```python
from build123d import *

# Parameters (mm, degrees)
SKETCH_W     = 20
SKETCH_H     = 10
SKETCH_R     = 1.25
PAD_DEPTH    = 6.5
SKETCH001_W  = 19
SKETCH001_H  = 4
PAD001_DEPTH = 0.1
SKETCH002_W  = 4
SKETCH002_H  = 0.1
PAD002_DEPTH = 5
FILLET_R     = 1.99
SKETCH003_R  = 2.5
PAD003_DEPTH = 3.8
SKETCH004_W  = 0.5
SKETCH004_H  = 3
PAD004_DEPTH = 4
FILLET001_R  = 1.49


with BuildPart() as part:
    # Sketch → Pad (new body)
    with BuildSketch(Plane.XZ):
        with Locations((10, 5)):
            Rectangle(SKETCH_W, SKETCH_H)
        with Locations((5, 2.5)):
            Circle(SKETCH_R, mode=Mode.SUBTRACT)
        with Locations((15, 2.5)):
            Circle(SKETCH_R, mode=Mode.SUBTRACT)
    extrude(amount=PAD_DEPTH)

    # Sketch001 (on Face3 of Pad) → Pad001 (join)
    with BuildSketch(Plane(origin=(2.5, 1.5, 10), x_dir=(-0.965926, 0, -0.258819), z_dir=(-0.258819, 0, 0.965926))):
        with Locations((-9.5, 4.728916)):
            Rectangle(SKETCH001_W, SKETCH001_H)
    extrude(amount=-PAD001_DEPTH)

    # Sketch002 (on Face12 of Pad001) → Pad002 (join)
    with BuildSketch(Plane(origin=(-2.332532, 0, 8.705127), x_dir=(-0.965926, 0, -0.258819), z_dir=(-0.258819, 0, 0.965926))):
        with Locations((-22.003005, 5.178916)):
            Rectangle(SKETCH002_W, SKETCH002_H)
        with Locations((-22.003005, 1.278916)):
            Rectangle(SKETCH002_W, SKETCH002_H)
    extrude(amount=PAD002_DEPTH)

    # Fillet
    fillet_edges = [part.edges().sort_by_distance(p)[0] for p in [
        (19.558495, -5.178916, 19.747191),
        (15.694792, -5.178916, 18.711915),
        (15.694792, -1.278916, 18.711915),
        (19.558495, -1.278916, 19.747191),
    ]]
    fillet(fillet_edges, radius=FILLET_R)

    # Sketch003 (on Face5 of Fillet) → Pad003 (join)
    with BuildSketch(Plane.XZ.offset(1.328916)):
        with Locations((18.132034, 17.304772)):
            Circle(SKETCH003_R)
    extrude(amount=PAD003_DEPTH)

    # Sketch004 (on Face24 of Pad003) → Pad004 (join)
    with BuildSketch(Plane(origin=(0, 0, 0), x_dir=(1, 0, 0), z_dir=(0, 0, -1))):
        with Locations((17.75, 3.25)):
            Rectangle(SKETCH004_W, SKETCH004_H)
        with Locations((11.25, 3.25)):
            Rectangle(SKETCH004_W, SKETCH004_H)
        with Locations((2.05, 3.25)):
            Rectangle(SKETCH004_W, SKETCH004_H)
    extrude(amount=PAD004_DEPTH)

    # Fillet001
    fillet001_edges = [part.edges().sort_by_distance(p)[0] for p in [
        (2.05, -4.75, -4),
        (2.05, -1.75, -4),
        (11.25, -4.75, -4),
        (11.25, -1.75, -4),
        (17.75, -4.75, -4),
        (17.75, -1.75, -4),
    ]]
    fillet(fillet001_edges, radius=FILLET001_R)


solid = part.part
```
Work out the finished part from the listing and answer in its coordinate system (mm). A direction names the side the tool comes from. Give positions to 0.01 mm unless a question says otherwise; leave off trailing zeros. Loops run counter-clockwise (first coordinate to the right, second up) from the corner with the lowest first, then second, coordinate; pieces in that order, holes last. Notation, with made-up numbers: (26, 63) -> (60, 63) arc R33 ccw to (60, 102) -> close; hole circle Ø10 at (88.25, -18). An arc over 180 degrees is marked (long way). One line per question, with ' | ' between items. Start each with the question number.
1) Section C-C, the plane z = 2.5 is taken. Determine the outline of the cut face in (x, y), then the cut area to 3 significant figures.
2) Section A-A, the plane x = 18.5 is taken. Determine the outline of the cut face in (y, z), then the cut area to 3 significant figures.
3) Straight lines are drawn through the part: L1, parallel to Z at x = 5, y = -0.25; L2, parallel to X at y = -3.5, z = 9; L3, parallel to X at y = -1.5, z = 1.75. For each, find the intervals that lie inside material, in ascending order.
4) Determine the mould class of faces 1 (the face through (2.053, -2.175, -3.552)), 2 (the face through (19, -1.229, 16)), 3 (the face through (14.079, -3.204, 3.345)) for opening direction Z: +Z half, -Z half, draft (parallel to the pull), parting line (faces both ways), or undercut.
5) Section B-B, the plane y = -2.75 is taken. Determine the outline of the cut face in (x, z).
6) Section D-D, the plane y = -6 is taken. Determine the outline of the cut face in (x, z), then the cut area to 3 significant figures.
7) For faces 4 (the face through (1.8, -3, -2)), 5 (the face through (20, -3, 5)), 6 (the face through (17, -5.229, 16)), 7 (the face through (2.3, -3, -2)), determine the directions among +Z, -Z, +X, -X, +Y, -Y from which every point of the face is accessible in a straight line to the end or side of a thin tool.
8) Each of these flat-tipped pins is pushed along its axis until it touches: pin 1 (4.5 mm diameter, centred on x = 14.5, z = 13.5, fed in from -Y); pin 2 (1.5 mm diameter, centred on y = -3, z = -3, fed in from -X); pin 3 (0.6 mm diameter, centred on x = 18, z = -0.5, fed in from +Y). Where does it stop, or does it pass through?
Resolved:
1) outline: (0, -6.5) -> (3.75, -6.5) -> (3.75, 0) -> (0, 0) -> close; (6.25, -6.5) -> (13.75, -6.5) -> (13.75, 0) -> (6.25, 0) -> close; (16.25, -6.5) -> (20, -6.5) -> (20, 0) -> (16.25, 0) -> close | area: 97.5 mm2
2) outline: (-6.5, 0) -> (0, 0) -> (0, 10) -> (-6.5, 10) -> close; (-5.23, 14.18) -> (-1.23, 14.18) -> (-1.23, 19.27) -> (-1.33, 19.27) -> (-1.33, 19.78) -> (-5.13, 19.78) -> (-5.13, 19.27) -> (-5.23, 19.27) -> close; hole (-5.13, 14.29) -> (-1.33, 14.29) -> (-1.33, 14.83) -> (-5.13, 14.83) -> close | area: 85.2 mm2
3) L1: 0 to 1.25, 3.75 to 10 | L2: 0 to 20 | L3: 0 to 4, 6 to 14, 16 to 20
4) face 1: -Z half | face 2: draft | face 3: undercut
5) outline: (0, 0) -> (1.8, 0) -> (1.8, -3.92) -> (2.3, -3.92) -> (2.3, 0) -> (11, 0) -> (11, -3.92) -> (11.5, -3.92) -> (11.5, 0) -> (17.5, 0) -> (17.5, -3.92) -> (18, -3.92) -> (18, 0) -> (20, 0) -> (20, 10) -> (2.89, 10) -> (20.88, 14.82) -> (20.85, 14.92) -> (2.5, 10) -> (0, 10) -> close; circle Ø5 at (18.13, 17.3); hole circle Ø2.5 at (5, 2.5); hole circle Ø2.5 at (15, 2.5)
6) outline: (0, 0) -> (20, 0) -> (20, 10) -> (0, 10) -> close; hole circle Ø2.5 at (5, 2.5); hole circle Ø2.5 at (15, 2.5) | area: 190 mm2
7) face 4: -Z, -X, +Y, -Y | face 5: -Z, +X, +Y, -Y | face 6: +Z, +X, -X, -Y | face 7: -Z, +Y, -Y
8) pin 1: y = -5.23 | pin 2: x = 1.8 | pin 3: y = -1.75
